Model file for the job. Use its own axes, mm. Face numbers are marked on the shaded views. Round coordinates to 2 decimals unless told otherwise and drop trailing zeros. Loops run counter-clockwise (first coordinate to the right, second up) from the corner with the lowest first, then second, coordinate; pieces in that order, holes last.
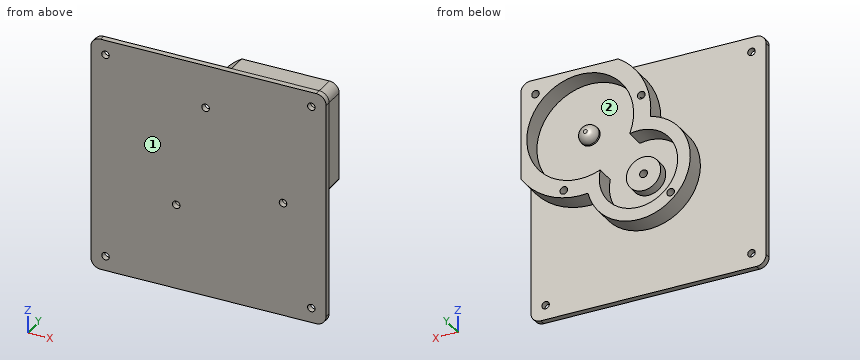
from build123d import *
from build123d.topology import SkipClean

# Parameters (mm, degrees)
SKETCH1_W                    = 152.4
SKETCH1_H                    = 3.81
MAIN_FRAME_DEPTH             = 152.4
FILLET1_R                    = 6.35
SKETCH3_R                    = 6.35
POT_GEAR_SNUB_NUB_DEPTH      = 6.35
SKETCH3_6_R                  = 11.1125
SKETCH3_6_R_2                = 2.54
BASE_SNUB_NUB_DEPTH          = 6.35
SKETCH7_R                    = 2.4384
CORNER_MOUNTING_HOLES_DEPTH  = 216.619670949
FILLET2_R                    = 5.08
F_10_0_1935_DIAMETER_HOLE1_D = 4.9149
BOSS_EXTRUDE2_OUTLINE_R      = 2.45745
BOSS_EXTRUDE2_OUTLINE_R_2    = 2.4384
BOSS_EXTRUDE2_DEPTH          = 12.794


# Read off the part's stored shape, not the designer's step: Boss-Extrude2
with BuildPart() as part:
    # Sketch1 → Main Frame (new body)
    with BuildSketch(Plane(origin=(0, 0, 0), x_dir=(0, 0, -1), z_dir=(1, 0, 0))):
        with Locations((76.2, -1.905)):
            Rectangle(SKETCH1_W, SKETCH1_H)
    extrude(amount=MAIN_FRAME_DEPTH)

    # Fillet1
    fillet1_edges = [part.edges().sort_by_distance(p)[0] for p in [
        (152.4, -1.905, -152.4),
        (152.4, -1.905, 0),
        (0, -1.905, -152.4),
        (0, -1.905, 0),
    ]]
    fillet(fillet1_edges, radius=FILLET1_R)

    # Sketch3 → Pot Gear Snub Nub (add)
    with BuildSketch(Plane(origin=(0, 0, 0), x_dir=(1, 0, 0), z_dir=(0, 1, 0))):
        with Locations(Location((113.917075708, 38.482924292, 0), (0, 0, 90))):
            Circle(SKETCH3_R)
    extrude(amount=POT_GEAR_SNUB_NUB_DEPTH)

    # Sketch3<6> → Base Snub Nub (add)
    with BuildSketch(Plane(origin=(0, 0, 0), x_dir=(1, 0, 0), z_dir=(0, 1, 0))):
        with Locations(Location((76.2, 76.2, 0), (0, 0, 90))):
            Circle(SKETCH3_6_R)
        with Locations(Location((76.2, 76.2, 0), (0, 0, 270))):
            Circle(SKETCH3_6_R_2, mode=Mode.SUBTRACT)
    extrude(amount=BASE_SNUB_NUB_DEPTH)

    # Sketch7 → Corner Mounting Holes (cut, through all)
    with BuildSketch(Plane(origin=(0, 0, 0), x_dir=(1, 0, 0), z_dir=(0, 1, 0))):
        with Locations(Location((142.875, 142.875, 0), (0, 0, 270))):
            Circle(SKETCH7_R)
        with Locations(Location((142.875, 9.525, 0), (0, 0, 270))):
            Circle(SKETCH7_R)
        with Locations(Location((9.525, 9.525, 0), (0, 0, 270))):
            Circle(SKETCH7_R)
        with Locations(Location((9.525, 142.875, 0), (0, 0, 270))):
            Circle(SKETCH7_R)
    extrude(amount=-CORNER_MOUNTING_HOLES_DEPTH, mode=Mode.SUBTRACT)

    # Fillet2
    fillet2_edges = [part.edges().sort_by_distance(p)[0] for p in [
        (113.917075708, 6.35, -32.132924292),
    ]]
    fillet(fillet2_edges, radius=FILLET2_R)

    # #10 (0.1935) Diameter Hole1 (through all)
    with Locations(Plane(origin=(0, 0, 0), x_dir=(1, 0, 0), z_dir=(0, 1, 0))):
        with Locations((124.51641164, 78.040184515), (74.359815485, 27.88358836), (55.344253184, 97.055746816)):
            Hole(F_10_0_1935_DIAMETER_HOLE1_D / 2)

    # Boss-Extrude2 outline → Boss-Extrude2 (add)
    with SkipClean():  # the faces are left unmerged after this step: merging them gives an invalid solid
        with BuildSketch(Plane(origin=(0, 0, 0), x_dir=(1, 0, 0), z_dir=(0, 1, 0))):
            with BuildLine():
                ThreePointArc((108.890253115, 83.92089943), (52.448527028, 99.951472972), (68.47910057, 43.509746885))
                ThreePointArc((68.47910057, 43.509746885), (72.658210549, 18.795756494), (89.240303876, 0))
                Line((89.240303876, 0), (146.05, 0))
                ThreePointArc((146.05, 0), (150.540128061, 1.859871939), (152.4, 6.35))
                Line((152.4, 6.35), (152.4, 63.159696124))
                ThreePointArc((152.4, 63.159696124), (133.604243506, 79.741789451), (108.890253115, 83.92089943))
            make_face()
            with Locations((74.359815485, 27.88358836)):
                Circle(BOSS_EXTRUDE2_OUTLINE_R, mode=Mode.SUBTRACT)
            with Locations((142.875, 9.525)):
                Circle(BOSS_EXTRUDE2_OUTLINE_R_2, mode=Mode.SUBTRACT)
            with BuildLine():
                ThreePointArc((81.82842228, 51.431454168), (58.239487758, 94.160512242), (100.968545832, 70.57157772))
                ThreePointArc((100.968545832, 70.57157772), (138.384871939, 14.015128061), (81.82842228, 51.431454168))
            make_face(mode=Mode.SUBTRACT)
            with Locations((55.344253184, 97.055746816)):
                Circle(BOSS_EXTRUDE2_OUTLINE_R, mode=Mode.SUBTRACT)
            with Locations((124.51641164, 78.040184515)):
                Circle(BOSS_EXTRUDE2_OUTLINE_R, mode=Mode.SUBTRACT)
        extrude(amount=BOSS_EXTRUDE2_DEPTH)


solid = part.part
Q1. Slice it at A-A on z = -142.5. Give the cut face in (x, y), plus the area to 3 significant figures.
Q2. Slice it at D-D on z = -114.5. Give the cut face in (x, y), plus the area to 3 significant figures.
Q3. Slice it at C-C on x = 94.5. Give the cut face in (y, z), plus the area to 3 significant figures.
Q4. Pull direction Z, two halves, no side cores. Call the marked faces 1 and 2: pulls with the +Z half, pulls with the -Z half, needs draft (parallel to the pull), parting line crosses it, or undercut.
Q5. Probe line 1 (Z direction, x = 144, y = 11.5); line 2 (X direction, y = 6.25, z = -8.5); line 3 (Y direction, x = 39, z = -22). List the from-to ranges inside material, lowest first.
Q6. Flat gauge pins, fed straight in: P1, Ø3, axis at x = 124.52, z = -78.04, coming from the -Y side; P2, Ø6, axis at y = 6, z = -61, coming from the -X side; P3, Ø3, axis at x = 67, y = 10, coming from the -Z side; P4, Ø11, axis at x = 81, z = -72.5, coming from the +Y side. Where does each tip first touch, or does it go through?
Reply:
1. outline: (0, -3.81) - (7.12, -3.81) - (7.12, 0) - (0, 0) - close; (11.93, -3.81) - (140.47, -3.81) - (140.47, 0) - (11.93, 0) - close; (145.28, -3.81) - (152.4, -3.81) - (152.4, 0) - (145.28, 0) - close
1. area: 544 mm2
2. outline: (0, -3.81) - (152.4, -3.81) - (152.4, 0) - (0, 0) - close
2. area: 581 mm2
3. outline: (-3.81, -152.4) - (0, -152.4) - (0, -104.37) - (12.79, -104.37) - (12.79, -93.81) - (0, -93.81) - (0, -9.84) - (12.79, -9.84) - (12.79, 0) - (-3.81, 0) - close
3. area: 842 mm2
4. face 1: needs draft
4. face 2: undercut
5. line 1: z = -72.91 to -55.58, -21.38 to -11.69, -7.36 to 0
5. line 2: x = 79.41 to 96.64, 131.19 to 140.66, 145.09 to 152.4
5. line 3: y = -3.81 to 0
6. P1: passes through
6. P2: stops at x = 44.9
6. P3: stops at z = -108.9
6. P4: stops at y = 6.35
